Geometry check sheet. Reference: the model listing, model coordinates, mm. A direction names the side the tool comes from. Coordinates: 2 decimals unless noted, no trailing zeros. Loops run counter-clockwise (first coordinate to the right, second up) from the corner with the lowest first, then second, coordinate; pieces in that order, holes last. Notation, with made-up numbers: M 43.25,19.5 L 64.25,19.5 A14 ccw 64.25,33.5 Z; hole C -16,85 d4. An arc over 180 degrees is marked long. Use CSV: the item, a comma, the result in double quotes.
```python
from build123d import *

# Parameters (mm, degrees)
EXTRUDE032_DEPTH = 5
SKETCH036_W      = 0.9
SKETCH036_H      = 1.25
EXTRUDE033_DEPTH = 7


with BuildPart() as extrude032:
    # Sketch035 → Extrude032 (new body)
    with BuildSketch(Plane.YZ.offset(67)):
        Polygon((60, 12.75), (62.15, 12.75), (62.15, 2.85), (64.85, 2.85), (64.85, 12.75), (67, 12.75), (67, 2), (60, 2), align=None)
    extrude(amount=EXTRUDE032_DEPTH)


with BuildPart() as obj1:
    # Sketch036 → Extrude033 (new body)
    with BuildSketch(Plane.XZ):
        with Locations((70.75, 2.625)):
            Rectangle(SKETCH036_W, SKETCH036_H)
    extrude(amount=EXTRUDE033_DEPTH)


with BuildPart() as obj1_1:
    # Extrude033 placement: moved
    add(obj1.part.moved(Location((0, 67, 0))))

    # Fusion: union Extrude032
    add(extrude032.part)


solid = obj1_1.part
```
1. Section check C-C, the plane y = 63.5. Record the cut outline in (x, z), plus the area to 3 significant figures.
The answers:
outline,"M 67,2 L 72,2 L 72,2.85 L 71.2,2.85 L 71.2,3.25 L 70.3,3.25 L 70.3,2.85 L 67,2.85 Z"
area,"4.61 mm^2"
2. Section check A-A, the plane z = 4.75. Record the cut outline in (x, y), plus the area to 3 significant figures.
The answers:
outline,"M 67,60 L 72,60 L 72,62.15 L 67,62.15 Z; M 67,64.85 L 72,64.85 L 72,67 L 67,67 Z"
area,"21.5 mm^2"
3. Set-up check for faces 4 (the flat face through (71, 64, 3.25)), 5 (the flat face through (69, 64, 2)), 6 (the flat face through (69, 63, 2.85)): record each of +Z, -Z, +X, -X, +Y, -Y from which the full face is reachable in a straight line by a thin tool's end or side.
The answers:
face 4,"+Z, +X, -X"
face 5,"-Z, +X, -X, +Y, -Y"
face 6,"+Z, -X"
4. Thickness scan on line 1 (Y direction, x = 67.5, z = 9); line 2 (Z direction, x = 69.85, y = 62.5); line 3 (Z direction, x = 70.4, y = 63.5). Record the ranges inside material, lowest first. Write a range as [from, to].
The answers:
line 1,"[60, 62.15], [64.85, 67]"
line 2,"[2, 2.85]"
line 3,"[2, 3.25]"
5. Release check for a two-part mould opening along Y. For faces 1 (the flat face through (69, 67, 7)), 2 (the flat face through (69, 60, 7)), 3 (the flat face through (69, 64.85, 8)) record: +Y half, -Y half, draft (parallel to the pull), parting line (faces both ways), or undercut.
The answers:
face 1,"+Y half"
face 2,"-Y half"
face 3,"undercut"
6. Section check B-B, the plane x = 69.9. Record the cut outline in (y, z), plus the area to 3 significant figures.
The answers:
outline,"M 60,2 L 67,2 L 67,12.75 L 64.85,12.75 L 64.85,2.85 L 62.15,2.85 L 62.15,12.75 L 60,12.75 Z"
area,"48.5 mm^2"
7. Gauge pin test, flat end, axial feed: P1, Ø0.7, axis at x = 70.5, y = 64, coming from the +Z side. Record the tip position at first contact, or that the pin passes through.
The answers:
P1,"z = 3.25"
